```python
from build123d import *

# Parameters (mm, degrees)
F1_DEPTH = 8
F2_W     = 30
F2_H     = 8
F3_DEPTH = 37
F4_W     = 30.001698
F4_H     = 8
F5_DEPTH = 37
F6_R     = 7.5
F7_DEPTH = 81.026
F8_R     = 7.5
F9_DEPTH = 57.15


with BuildPart() as f1:
    # F0 (on Front) → F1 (new body)
    with BuildSketch(Plane.XZ):
        Polygon((-26.677133, 36.321553), (-56.675435, 36.002424), (-56.675435, -8.997576), (33.324565, -8.997576), (33.324565, 36.321553), (3.322867, 36.321553), (-26.677133, 16.321553), align=None)
    extrude(amount=F1_DEPTH)

    # F2 (on face) → F3 (join)
    with BuildSketch(Plane.XZ.offset(8)):
        with Locations((18.324565, -4.997576)):
            Rectangle(F2_W, F2_H)
    extrude(amount=F3_DEPTH)

    # F4 (on face) → F5 (join)
    with BuildSketch(Plane.XZ.offset(8)):
        with Locations((18.323716, 32.321553)):
            Rectangle(F4_W, F4_H)
    extrude(amount=F5_DEPTH)

    # F6 (on face) → F7 (cut)
    with BuildSketch(Plane.XY.offset(36.321553)):
        with Locations((18.322867, -22.5)):
            Circle(F6_R)
    extrude(amount=-F7_DEPTH, mode=Mode.SUBTRACT)

    # F8 (on face) → F9 (cut)
    with BuildSketch(Plane.XZ.offset(8)):
        with Locations((-41.675435, 13.661989)):
            Circle(F8_R)
    extrude(amount=-F9_DEPTH, mode=Mode.SUBTRACT)


solid = f1.part
```
Here's how the part is built. I have some questions about the finished solid (model axes, mm). A direction names the side the tool comes from. Give positions to 0.01 mm unless a question says otherwise; leave off trailing zeros. Order: outer loops, then holes, each group sorted by start corner. A loop starts at its lowest first (then second) coordinate and runs counter-clockwise, first axis right, second up. Notation, with made-up numbers: (40.5, -36) - (87.5, -36) arc R19 ccw to (87.5, -18) - close; hole circle Ø10 at (-35, -15.75). An arc over 180 degrees is marked (long way). Answer as a JSON object with one key per item and string values. Group by question number.
Item 1: If we section it at D-D on z = 8.5: Please give me the cut outline in (x, y), and give its area (3 significant figures).
Item 2: If we section it at A-A on y = -22.5: Please give me the cut outline in (x, z), and give its area (3 significant figures).
Item 3: Which directions (+Z, -Z, +X, -X, +Y, -Y) give clear straight access to the entire face, cutting with the end or side of a thin tool? Please do faces 1 (the flat face through (-56.675, -4, 14)), 2 (the flat face through (-26.677, -4, 26)), 3 (the flat face through (18.1, -30.4, -0.998)), 4 (the flat face through (3.325, -26, -5)).
Item 4: If we mould it in two halves opening along Y, with no side actions, what happens to faces 5 (the cylindrical face through (12.795, -17.431, 32.378)), 6 (the flat face through (18, -45, 32)), 7 (the cylindrical face through (12.795, -17.431, -4.942)), 8 (the flat face through (3.323, -26, 32))? For each: pulls with the +Y half, pulls with the -Y half, needs draft (parallel to the pull), parting line crosses it, or undercut.
Item 5: Please list where these lines run through material, in increasing order: probe 1 along Z at (x, y) = (22, -36); probe 2 along Y at (x, z) = (-51.5, 29.5); probe 3 along Y at (x, z) = (25, 34).
Item 6: For P1, Ø6, axis at y = -26.5, z = -4, coming from the -X side, with a flat end and sliding along its axis, tell me the tip position at first contact or that it passes through.
Item 7: If we section it at B-B on z = -3: Please give me the cut outline in (x, y), and give its area (3 significant figures).
Item 8: If we section it at C-C on x = 8.5: Please give me the cut outline in (y, z), and give its area (3 significant figures).
Result set:
{
 "1": {"outline": "(-56.68, -8) - (-47.12, -8) - (-47.12, 0) - (-56.68, 0) - close; (-36.23, -8) - (33.32, -8) - (33.32, 0) - (-36.23, 0) - close", "area": "633 mm²"},
 "2": {"outline": "(3.32, -9) - (10.82, -9) - (10.82, -1) - (3.32, -1) - close; (3.32, 28.32) - (10.82, 28.32) - (10.82, 36.32) - (3.32, 36.32) - close; (25.82, -9) - (33.32, -9) - (33.32, -1) - (25.82, -1) - close; (25.82, 28.32) - (33.32, 28.32) - (33.32, 36.32) - (25.82, 36.32) - close", "area": "240 mm²"},
 "3": {"face 1": "+Z, -Z, -X, +Y, -Y", "face 2": "+Z, +Y, -Y", "face 3": "+X, -X, -Y", "face 4": "+Z, -Z, -X, -Y"},
 "4": {"face 5": "undercut", "face 6": "pulls with the -Y half", "face 7": "undercut", "face 8": "needs draft"},
 "5": {"probe 1": "-9 to -1, 28.32 to 36.32", "probe 2": "-8 to 0", "probe 3": "-45 to -25.92, -19.08 to 0"},
 "6": {"P1": "x = 3.32"},
 "7": {"outline": "(-56.68, -8) - (3.32, -8) - (3.32, -45) - (33.32, -45) - (33.32, 0) - (-56.68, 0) - close; hole circle Ø15 at (18.32, -22.5)", "area": "1,650 mm²"},
 "8": {"outline": "(-45, -9) - (0, -9) - (0, 36.32) - (-45, 36.32) - (-45, 28.32) - (-8, 28.32) - (-8, -1) - (-45, -1) - close", "area": "955 mm²"}
}
